Design review of the part built by this model. Coordinates are the model's own, in mm. A direction names the side the tool comes from. Give positions to 0.01 mm unless a question says otherwise; leave off trailing zeros. Write each loop counter-clockwise with the first axis right and the second up, starting at its lowest first coordinate (ties: lowest second). Pieces come first, ordered by that corner, then holes.
```python
from build123d import *

# Parameters (mm, degrees)
SALIENTE_EXTRUIR1_DEPTH    = 4
CROQUIS2_W                 = 55
CROQUIS2_H                 = 101
CORTAR_EXTRUIR1_DEPTH      = 2
CROQUIS12_W                = 3
CROQUIS12_H                = 11
SALIENTE_EXTRUIR2_DEPTH    = 15
CROQUIS13_W                = 5
CROQUIS13_H                = 12
CORTAR_EXTRUIR8_DEPTH      = 80
CORTAR_EXTRUIR8_DEPTH_BACK = 4
CROQUIS14_W                = 5
CROQUIS14_H                = 12
CORTAR_EXTRUIR9_DEPTH      = 80
CORTAR_EXTRUIR9_DEPTH_BACK = 4
CROQUIS15_W                = 35
CROQUIS15_H                = 10
CORTAR_EXTRUIR10_DEPTH     = 20


with BuildPart() as part:
    # Croquis1 → Saliente-Extruir1 (new body)
    with BuildSketch(Plane(origin=(0, 0, 0), x_dir=(1, 0, 0), z_dir=(0, 1, 0))):
        Polygon((30, -52.5), (30, -22.5), (41, -22.5), (41, -11.5), (30, -11.5), (30, 11.5), (41, 11.5), (41, 22.5), (30, 22.5), (30, 52.5), (-30, 52.5), (-30, 22.5), (-41, 22.5), (-41, 11.5), (-30, 11.5), (-30, -11.5), (-41, -11.5), (-41, -22.5), (-30, -22.5), (-30, -52.5), align=None)
    extrude(amount=SALIENTE_EXTRUIR1_DEPTH)

    # Croquis2 → Cortar-Extruir1 (cut)
    with BuildSketch(Plane(origin=(0, 4, 0), x_dir=(1, 0, 0), z_dir=(0, 1, 0))):
        Rectangle(CROQUIS2_W, CROQUIS2_H)
    extrude(amount=-CORTAR_EXTRUIR1_DEPTH, mode=Mode.SUBTRACT)

    # Croquis12 → Saliente-Extruir2 (add)
    with BuildSketch(Plane(origin=(0, 4, 0), x_dir=(1, 0, 0), z_dir=(0, 1, 0))):
        with Locations((-39.5, 17)):
            Rectangle(CROQUIS12_W, CROQUIS12_H)
        with Locations((-39.5, -17)):
            Rectangle(CROQUIS12_W, CROQUIS12_H)
        with Locations((39.5, -17)):
            Rectangle(CROQUIS12_W, CROQUIS12_H)
        with Locations((39.5, 17)):
            Rectangle(CROQUIS12_W, CROQUIS12_H)
    extrude(amount=SALIENTE_EXTRUIR2_DEPTH)

    # Croquis13 → Cortar-Extruir8 (cut, two sides)
    with BuildSketch(Plane.ZY.offset(-38)) as cortar_extruir8_sk:
        with Locations((-17, 10)):
            Rectangle(CROQUIS13_W, CROQUIS13_H)
    extrude(amount=CORTAR_EXTRUIR8_DEPTH, mode=Mode.SUBTRACT)
    extrude(cortar_extruir8_sk.sketch, amount=-CORTAR_EXTRUIR8_DEPTH_BACK, mode=Mode.SUBTRACT)

    # Croquis14 → Cortar-Extruir9 (cut, two sides)
    with BuildSketch(Plane.ZY.offset(-38)) as cortar_extruir9_sk:
        with Locations((17, 10)):
            Rectangle(CROQUIS14_W, CROQUIS14_H)
    extrude(amount=CORTAR_EXTRUIR9_DEPTH, mode=Mode.SUBTRACT)
    extrude(cortar_extruir9_sk.sketch, amount=-CORTAR_EXTRUIR9_DEPTH_BACK, mode=Mode.SUBTRACT)

    # Croquis15 → Cortar-Extruir10 (cut, through all)
    with BuildSketch(Plane(origin=(0, 0, 0), x_dir=(1, 0, 0), z_dir=(0, 1, 0))):
        Rectangle(CROQUIS15_W, CROQUIS15_H)
        with Locations((0, -18)):
            Rectangle(CROQUIS15_W, CROQUIS15_H)
        with Locations((0, -36)):
            Rectangle(CROQUIS15_W, CROQUIS15_H)
        with Locations((0, 18)):
            Rectangle(CROQUIS15_W, CROQUIS15_H)
        with Locations((0, 36)):
            Rectangle(CROQUIS15_W, CROQUIS15_H)
    extrude(amount=CORTAR_EXTRUIR10_DEPTH, mode=Mode.SUBTRACT)


solid = part.part
```
(1) Consider section D-D, the plane z = 43.5. Give the boundary of the cut face in (x, y), then the cut area to 3 significant figures.
Resolved:
outline: (-30, 0) - (30, 0) - (30, 4) - (27.5, 4) - (27.5, 2) - (-27.5, 2) - (-27.5, 4) - (-30, 4) - close
area: 130 mm2
(2) Mouldability with a two-part tool opening along Z and no side actions: class faces 4 (the face through (-39, 7, -22.5)), 5 (the face through (-39, 5, 11.5)), 6 (the face through (38, 13, -14)), 7 (the face through (-39, 10, -14.5)) as pulls with the +Z half, pulls with the -Z half, needs draft (parallel to the pull), parting line crosses it, or undercut.
Resolved:
face 4: pulls with the -Z half
face 5: undercut
face 6: needs draft
face 7: undercut
(3) Consider section B-B, the plane y = 13.5. Give the number of separate pieces and of enclosed holes in the cut face, then the cut area to 3 significant figures.
Resolved:
separate pieces: 8
enclosed holes: 0
area: 72.0 mm2
(4) Tool access review of faces 1 (the face through (0, 2, -12)), 2 (the face through (-30, 2, -38)), 3 (the face through (39, 10, -14.5)): name each direction out of +Z, -Z, +X, -X, +Y, -Y from which nothing blocks a thin tool from reaching the whole face with its end or side.
Resolved:
face 1: +Y
face 2: -Z, -X, +Y, -Y
face 3: +X, -X
(5) Consider section A-A, the plane z = 1. Give the boundary of the cut face in (x, y).
Resolved:
outline: (-30, 0) - (-17.5, 0) - (-17.5, 2) - (-27.5, 2) - (-27.5, 4) - (-30, 4) - close; (17.5, 0) - (30, 0) - (30, 4) - (27.5, 4) - (27.5, 2) - (17.5, 2) - close
(6) Clearance check with flat-ended pins moving along their axes: P1, Ø5, axis at y = 3, z = -42, coming from the -X side; P2, Ø2.5, axis at x = 39.5, y = 12.5, coming from the +Z side; P3, Ø2, axis at x = 8.5, y = 4.5, coming from the -Z side; P4, Ø1.5, axis at x = 39.5, y = 11, coming from the -Z side. State where each tip first meets the part, or that it passes through.
Resolved:
P1: stops at x = -30
P2: stops at z = 22.5
P3: stops at z = -52.5
P4: stops at z = -22.5
(7) To check wall thickness, follow L1, parallel to X at y = 2.25, z = 27; L2, parallel to X at y = 7.25, z = -14; L3, parallel to Z at x = 15, y = 3.25. State the ranges of each line that lie inside material, in increasing order.
Resolved:
L1: x = -30 to -27.5, 27.5 to 30
L2: x = -41 to -38, 38 to 41
L3: z = -52.5 to -50.5, 50.5 to 52.5
(8) Consider section C-C, the plane x = -33. Give the boundary of the cut face in (y, z), then the cut area to 3 significant figures.
Resolved:
outline: (0, -22.5) - (4, -22.5) - (4, -11.5) - (0, -11.5) - close; (0, 11.5) - (4, 11.5) - (4, 22.5) - (0, 22.5) - close
area: 88.0 mm2
